Check sheet for the modelled part. Datum: model origin and axes. Units: mm. A direction names the side the tool comes from. Round coordinates to 2 decimals unless told otherwise and drop trailing zeros. Write each loop counter-clockwise with the first axis right and the second up, starting at its lowest first coordinate (ties: lowest second). Pieces come first, ordered by that corner, then holes. Notation, with made-up numbers: (-33, 30) -> (-23, 30) arc R19 cw to (-23, 36) -> close; hole circle Ø6 at (22, 72.25). An arc over 180 degrees is marked (long way). One line per item, written item: value. Start each with the question number.
```python
from build123d import *

# Parameters (mm, degrees)
SKICA1_W                = 300
SKICA1_H                = 300
P_IDAT_VYSUNUT_M1_DEPTH = 10
P_IDAT_VYSUNUT_M3_DEPTH = 10


with BuildPart() as part:
    # Skica1 → Přidat vysunutím1 (new body)
    with BuildSketch(Plane.XY):
        with Locations((150, 150)):
            Rectangle(SKICA1_W, SKICA1_H)
    extrude(amount=P_IDAT_VYSUNUT_M1_DEPTH)

    # Skica3 → Přidat vysunutím3 (add)
    with BuildSketch(Plane.XY.offset(10)):
        with BuildLine():
            ThreePointArc((68.888397272, 112.33931183), (64.495171116, 77.345400758), (93.328139617, 57.034463419))
            ThreePointArc((93.328139617, 57.034463419), (82.601051267, 79.285579191), (89.763558517, 102.926244737))
            ThreePointArc((89.763558517, 102.926244737), (94.156784672, 137.920155809), (65.323816172, 158.231093148))
            ThreePointArc((65.323816172, 158.231093148), (76.050904522, 135.979977376), (68.888397272, 112.33931183))
        make_face()
        with BuildLine():
            ThreePointArc((109.948101695, 63.283359984), (105.735567111, 28.267237976), (134.672993338, 8.105402458))
            ThreePointArc((134.672993338, 8.105402458), (123.831191153, 30.300850255), (130.871573598, 53.978172582))
            ThreePointArc((130.871573598, 53.978172582), (135.084108182, 88.994294591), (106.146681955, 109.156130109))
            ThreePointArc((106.146681955, 109.156130109), (116.98848414, 86.960682312), (109.948101695, 63.283359984))
        make_face()
        with BuildLine():
            ThreePointArc((133.307752162, 149.58869496), (124.467578103, 115.44597142), (150.460873085, 91.608545718))
            ThreePointArc((150.460873085, 91.608545718), (142.672820518, 115.050576661), (152.804965779, 137.578830254))
            ThreePointArc((152.804965779, 137.578830254), (161.645139837, 171.721553795), (135.651844855, 195.558979497))
            ThreePointArc((135.651844855, 195.558979497), (143.439897423, 172.116948553), (133.307752162, 149.58869496))
        make_face()
        with BuildLine():
            ThreePointArc((246.236441483, 102.926244737), (241.843215328, 137.920155809), (270.676183828, 158.231093148))
            ThreePointArc((270.676183828, 158.231093148), (259.949095478, 135.979977376), (267.111602728, 112.33931183))
            ThreePointArc((267.111602728, 112.33931183), (271.504828884, 77.345400758), (242.671860383, 57.034463419))
            ThreePointArc((242.671860383, 57.034463419), (253.398948733, 79.285579191), (246.236441483, 102.926244737))
        make_face()
        with BuildLine():
            ThreePointArc((226.051898305, 63.283359984), (230.264432889, 28.267237976), (201.327006662, 8.105402458))
            ThreePointArc((201.327006662, 8.105402458), (212.168808847, 30.300850255), (205.128426402, 53.978172582))
            ThreePointArc((205.128426402, 53.978172582), (200.915891818, 88.994294591), (229.853318045, 109.156130109))
            ThreePointArc((229.853318045, 109.156130109), (219.01151586, 86.960682312), (226.051898305, 63.283359984))
        make_face()
        with BuildLine():
            ThreePointArc((202.692247838, 149.58869496), (211.532421897, 115.44597142), (185.539126915, 91.608545718))
            ThreePointArc((185.539126915, 91.608545718), (193.327179482, 115.050576661), (183.195034221, 137.578830254))
            ThreePointArc((183.195034221, 137.578830254), (174.354860163, 171.721553795), (200.348155145, 195.558979497))
            ThreePointArc((200.348155145, 195.558979497), (192.560102577, 172.116948553), (202.692247838, 149.58869496))
        make_face()
    extrude(amount=P_IDAT_VYSUNUT_M3_DEPTH)


solid = part.part
```
1. Release check for a two-part mould opening along X. For faces 4 (the face through (300, 148, 5)), 5 (the face through (123.862, 29.948, 14.93)), 6 (the face through (193, 144, 20)), 7 (the face through (174.21, 171.22, 14.93)) record: +X half, -X half, draft (parallel to the pull), parting line (faces both ways), or undercut.
2. Cross-section at C-C (y = 76). Record the cut outline in (x, z), plus the area to 3 significant figures.
3. Material ranges on probe 1 along X at (y, z) = (91.5, 15); probe 2 along X at (y, z) = (151.5, 11.25); probe 3 along X at (y, z) = (96.5, 11), recorded low to high.
4. Cross-section at B-B (z = 16.25). Record the cut outline in (x, y).
5. Cross-section at A-A (y = 41). Record the cut outline in (x, z).
6. Cross-section at D-D (y = 266.5). Record the cut outline in (x, z).
7. Depth check by flat-ended pin: pin 1 Ø3 at (x, y) = (38.5, 242.5) entering from +Z; pin 2 Ø1 at (x, z) = (127.5, 13) entering from +Y; pin 3 Ø5 at (x, z) = (269, 15.5) entering from -Y. Enter the tip coordinate at first touch or a pass-through.
8. Access from +Z, -Z, +X, -X, +Y, -Y to the whole of each face (thin tool, end or side, straight path). Record for faces 1 (the face through (64.3, 77.8, 14.9)), 2 (the face through (79, 108, 20)), 3 (the face through (135.3, 88.5, 14.9)).
Working result:
1. face 4: +X half
1. face 5: undercut
1. face 6: draft
1. face 7: undercut
2. outline: (0, 0) -> (300, 0) -> (300, 10) -> (270.88, 10) -> (270.88, 20) -> (252.98, 20) -> (252.98, 10) -> (219.89, 10) -> (219.89, 20) -> (197.94, 20) -> (197.94, 10) -> (138.06, 10) -> (138.06, 20) -> (116.11, 20) -> (116.11, 10) -> (83.02, 10) -> (83.02, 20) -> (65.12, 20) -> (65.12, 10) -> (0, 10) -> close
2. area: 3,800 mm^2
3. probe 1: x = 61.57 to 83.88, 116.3 to 133.84, 202.16 to 219.7, 252.12 to 274.43
3. probe 2: x = 70.9 to 83.35, 135.11 to 161.4, 174.6 to 200.89, 252.65 to 265.1
3. probe 3: x = 61.99 to 85.78, 114.78 to 130.48, 138.56 to 147.08, 188.92 to 197.44, 205.52 to 221.22, 250.22 to 274.01
4. outline: (65.32, 158.23) arc R34.01 cw to (68.89, 112.34) arc R34.24 ccw to (93.33, 57.03) arc R34.01 cw to (89.76, 102.93) arc R34.24 ccw to start; (106.15, 109.16) arc R34.01 cw to (109.95, 63.28) arc R34.24 ccw to (134.67, 8.11) arc R34.01 cw to (130.87, 53.98) arc R34.24 ccw to start; (133.31, 149.59) arc R34.24 ccw to (150.46, 91.61) arc R34.01 cw to (152.8, 137.58) arc R34.24 ccw to (135.65, 195.56) arc R34.01 cw to start; (183.2, 137.58) arc R34.01 cw to (185.54, 91.61) arc R34.24 ccw to (202.69, 149.59) arc R34.01 cw to (200.35, 195.56) arc R34.24 ccw to start; (201.33, 8.11) arc R34.24 ccw to (226.05, 63.28) arc R34.01 cw to (229.85, 109.16) arc R34.24 ccw to (205.13, 53.98) arc R34.01 cw to start; (242.67, 57.03) arc R34.24 ccw to (267.11, 112.34) arc R34.01 cw to (270.68, 158.23) arc R34.24 ccw to (246.24, 102.93) arc R34.01 cw to start
5. outline: (0, 0) -> (300, 0) -> (300, 10) -> (233.23, 10) -> (233.23, 20) -> (211.36, 20) -> (211.36, 10) -> (124.64, 10) -> (124.64, 20) -> (102.77, 20) -> (102.77, 10) -> (0, 10) -> close
6. outline: (0, 0) -> (300, 0) -> (300, 10) -> (0, 10) -> close
7. pin 1: stops at z = 10
7. pin 2: stops at y = 142.88
7. pin 3: stops at y = 69.28
8. face 1: +Z, -X
8. face 2: +Z, +X, -X, +Y, -Y
8. face 3: +Z
